For this review, take the finished solid that the model builds, in its own axes (mm). Round coordinates to 2 decimals unless told otherwise and drop trailing zeros. Write each loop counter-clockwise with the first axis right and the second up, starting at its lowest first coordinate (ties: lowest second). Pieces come first, ordered by that corner, then holes. Notation, with made-up numbers: (71, 36.5) -> (86, 36.5) arc R16 ccw to (86, 56.5) -> close; hole circle Ø7 at (63.25, 11.25). An arc over 180 degrees is marked (long way). Answer in a Markdown table with one row per item.
from build123d import *

# Parameters (mm, degrees)
F0_R     = 3.175
F1_DEPTH = 6.35


with BuildPart() as f1:
    # F0 (on Top) → F1 (new body)
    with BuildSketch(Plane.XY):
        Polygon((-31.75, 50.8), (-50.8, 50.8), (-50.8, -50.8), (50.8, -50.8), (50.8, -31.75), (-31.75, -31.75), align=None)
        with Locations((-15.875, -41.275)):
            Circle(F0_R, mode=Mode.SUBTRACT)
        with Locations((-41.275, -15.143792145)):
            Circle(F0_R, mode=Mode.SUBTRACT)
        with Locations((41.275, -41.275)):
            Circle(F0_R, mode=Mode.SUBTRACT)
        with Locations((-41.275, 42.006207855)):
            Circle(F0_R, mode=Mode.SUBTRACT)
    extrude(amount=F1_DEPTH)


solid = f1.part
1) Consider section A-A on y = -43. State the section outline as (x, z) points, then the cut area to 3 significant figures.
Solved:
| item | result |
|---|---|
| outline | (-50.8, 0) -> (-18.54, 0) -> (-18.54, 6.35) -> (-50.8, 6.35) -> close; (-13.21, 0) -> (38.61, 0) -> (38.61, 6.35) -> (-13.21, 6.35) -> close; (43.94, 0) -> (50.8, 0) -> (50.8, 6.35) -> (43.94, 6.35) -> close |
| area | 577 mm² |
2) Consider section C-C on z = 3. State the section outline as (x, y) points (3 decimals).
Solved:
| item | result |
|---|---|
| outline | (-50.8, -50.8) -> (50.8, -50.8) -> (50.8, -31.75) -> (-31.75, -31.75) -> (-31.75, 50.8) -> (-50.8, 50.8) -> close; hole circle Ø6.35 at (-41.275, -15.144); hole circle Ø6.35 at (-41.275, 42.006); hole circle Ø6.35 at (-15.875, -41.275); hole circle Ø6.35 at (41.275, -41.275) |
3) Clearance check with a flat-ended pin moving along its axis: pin 1 Ø4 at (x, y) = (-41.28, -15.14) entering from +Z. State where the tip first meets the part, or that it passes through.
Solved:
| item | result |
|---|---|
| pin 1 | through |
4) Mouldability with a two-part tool opening along X and no side actions: class faces 1 (the flat face through (-31.75, 9, 3)), 2 (the cylindrical face through (-41.963, 38.907, 3.131)), 3 (the flat face through (10, -31.75, 3)), 4 (the flat face through (-50.8, 1, 3)) as pulls with the +X half, pulls with the -X half, needs draft (parallel to the pull), parting line crosses it, or undercut.
Solved:
| item | result |
|---|---|
| face 1 | pulls with the +X half |
| face 2 | undercut |
| face 3 | needs draft |
| face 4 | pulls with the -X half |
5) Consider section D-D on y = 14.5. State the section outline as (x, z) points.
Solved:
| item | result |
|---|---|
| outline | (-50.8, 0) -> (-31.75, 0) -> (-31.75, 6.35) -> (-50.8, 6.35) -> close |
6) For line 1 (Y direction, x = -15.5, z = 3); line 2 (X direction, y = -38.5, z = 4.75); line 3 (Y direction, x = -44, z = 6), list the stretches that pass through material, from the lowest coordinate up. Write a range as [from, to].
Solved:
| item | result |
|---|---|
| line 1 | [-50.8, -44.43], [-38.12, -31.75] |
| line 2 | [-50.8, -17.42], [-14.33, 39.73], [42.82, 50.8] |
| line 3 | [-50.8, -16.77], [-13.51, 40.38], [43.64, 50.8] |
7) Consider section B-B on x = -17. State the section outline as (y, z) points, then the cut area to 3 significant figures.
Solved:
| item | result |
|---|---|
| outline | (-50.8, 0) -> (-44.24, 0) -> (-44.24, 6.35) -> (-50.8, 6.35) -> close; (-38.31, 0) -> (-31.75, 0) -> (-31.75, 6.35) -> (-38.31, 6.35) -> close |
| area | 83.3 mm² |
